from build123d import *

# Parameters (mm, degrees)
SKETCH1_W           = 54
SKETCH1_H           = 59
SKETCH1_W_2         = 40
SKETCH1_H_2         = 52
BOSS_EXTRUDE1_DEPTH = 12
SKETCH2_R           = 1.85
CUT_EXTRUDE1_DEPTH  = 10
SKETCH3_R           = 1.85
CUT_EXTRUDE2_DEPTH  = 10
SKETCH4_W           = 54
SKETCH4_H           = 12
CUT_EXTRUDE4_DEPTH  = 40
SKETCH5_W           = 7
SKETCH5_H           = 12
CUT_EXTRUDE5_DEPTH  = 40
SKETCH6_W           = 12
SKETCH6_H           = 12
BOSS_EXTRUDE2_DEPTH = 5
SKETCH7_R           = 2.6
CUT_EXTRUDE6_DEPTH  = 2.4


with BuildPart() as part:
    # Sketch1 → Boss-Extrude1 (new body)
    with BuildSketch(Plane.XY):
        with Locations((27, 29.5)):
            Rectangle(SKETCH1_W, SKETCH1_H)
        with Locations((27, 29.5)):
            Rectangle(SKETCH1_W_2, SKETCH1_H_2, mode=Mode.SUBTRACT)
    extrude(amount=BOSS_EXTRUDE1_DEPTH)

    # Sketch2 → Cut-Extrude1 (cut)
    with BuildSketch(Plane(origin=(0, 59, 0), x_dir=(1, 0, 0), z_dir=(0, 1, 0))):
        with Locations(Location((13, -9.7, 0), (0, 0, 180))):
            Circle(SKETCH2_R)
        with Locations(Location((41, -9.7, 0), (0, 0, 180))):
            Circle(SKETCH2_R)
        with Locations(Location((27, -9.7, 0), (0, 0, 180))):
            Circle(SKETCH2_R)
    extrude(amount=-CUT_EXTRUDE1_DEPTH, mode=Mode.SUBTRACT)

    # Sketch3 → Cut-Extrude2 (cut)
    with BuildSketch(Plane.XZ):
        with Locations(Location((12.75, 6, 0), (0, 0, 270))):
            Circle(SKETCH3_R)
        with Locations(Location((41.25, 6, 0), (0, 0, 90))):
            Circle(SKETCH3_R)
    extrude(amount=-CUT_EXTRUDE2_DEPTH, mode=Mode.SUBTRACT)

    # Sketch4 → Cut-Extrude4 (cut)
    with BuildSketch(Plane.XZ):
        with Locations((27, 6)):
            Rectangle(SKETCH4_W, SKETCH4_H)
    extrude(amount=-CUT_EXTRUDE4_DEPTH, mode=Mode.SUBTRACT)

    # Sketch5 → Cut-Extrude5 (cut)
    with BuildSketch(Plane.XZ.offset(-40)):
        with Locations((3.5, 6)):
            Rectangle(SKETCH5_W, SKETCH5_H)
        with Locations((50.5, 6)):
            Rectangle(SKETCH5_W, SKETCH5_H)
    extrude(amount=-CUT_EXTRUDE5_DEPTH, mode=Mode.SUBTRACT)

    # Sketch6 → Boss-Extrude2 (add)
    with BuildSketch(Plane(origin=(47, 0, 0), x_dir=(0, 0, -1), z_dir=(1, 0, 0))):
        with Locations((-6, 53)):
            Rectangle(SKETCH6_W, SKETCH6_H)
    boss_extrude2 = extrude(amount=BOSS_EXTRUDE2_DEPTH)

    # Mirror1: Boss-Extrude2 across plane
    add(boss_extrude2.mirror(Plane.ZY.offset(-27)))

    # Sketch7 → Cut-Extrude6 (cut)
    with BuildSketch(Plane.ZY.offset(-2)):
        with Locations((6, 54)):
            Circle(SKETCH7_R)
    cut_extrude6 = extrude(amount=-CUT_EXTRUDE6_DEPTH, mode=Mode.SUBTRACT)

    # Mirror2: Cut-Extrude6 across plane
    add(cut_extrude6.mirror(Plane.ZY.offset(-27)), mode=Mode.SUBTRACT)


solid = part.part
For this review, take the finished solid that the model builds, in its own axes (mm). A direction names the side the tool comes from. Round coordinates to 2 decimals unless told otherwise and drop trailing zeros. Order: outer loops, then holes, each group sorted by start corner. A loop starts at its lowest first (then second) coordinate and runs counter-clockwise, first axis right, second up. Notation, with made-up numbers: M -38,49 L 3,49 A31 ccw 3,79 Z; hole C -22,16 d7. An arc over 180 degrees is marked long. Use a Markdown table: item, result. Add a question column.
Item 1: Add section A-A, the plane z = 9.7. Give the boundary of the cut face in (x, y), then the cut area to 3 significant figures.
Item 2: Add section D-D, the plane z = 1.5. Give the boundary of the cut face in (x, y), then the cut area to 3 significant figures.
Item 3: Tool access review of faces 4 (the cylindrical face through (50.82, 51.46, 5.44)), 5 (the flat face through (7, 51, 6)), 6 (the flat face through (4.4, 54, 6)): name each direction out of +Z, -Z, +X, -X, +Y, -Y from which nothing blocks a thin tool from reaching the whole face with its end or side.
Item 4: Insertion check: pin 1 (3 mm diameter, centred on x = 27, z = 9.7, fed in from +Y); pin 2 (1.6 mm diameter, centred on y = 55, z = 7, fed in from -X). Each pin has a flat end and moves straight along its axis. Give the tip position at first contact, or say it passes through.
Item 5: To check wall thickness, follow line 1 along X through (y, z) = (55, 7.25); line 2 along X through (y, z) = (52.5, 9.5); line 3 along Y through (x, z) = (50.95, 6). State the ranges of each line that lie inside material, in increasing order.
Item 6: Add section B-B, the plane x = 41. Give the boundary of the cut face in (y, z).
Item 7: Mouldability with a two-part tool opening along Y and no side actions: class faces 1 (the flat face through (27, 56, 12)), 2 (the flat face through (5, 47, 6)), 3 (the flat face through (49.6, 54, 6)) as released by +Y, released by -Y, zero draft, split by the parting line, or undercut.
Item 8: Add section C-C, the plane y = 49. Give the boundary of the cut face in (x, z).
Geometry results:
| question | item | result |
|---|---|---|
| 1 | outline | M 2,47 L 7,47 L 7,55.5 L 11.15,55.5 L 11.15,59 L 2,59 Z; M 14.85,55.5 L 25.15,55.5 L 25.15,59 L 14.85,59 Z; M 28.85,55.5 L 39.15,55.5 L 39.15,59 L 28.85,59 Z; M 42.85,55.5 L 47,55.5 L 47,47 L 52,47 L 52,59 L 42.85,59 Z |
| 1 | area | 221 mm² |
| 2 | outline | M 2,47 L 7,47 L 7,55.5 L 47,55.5 L 47,47 L 52,47 L 52,59 L 2,59 Z |
| 2 | area | 260 mm² |
| 3 | face 4 | +X |
| 3 | face 5 | +Z, -Z, -Y |
| 3 | face 6 | -X |
| 4 | pin 1 | passes through |
| 4 | pin 2 | stops at x = 4.4 |
| 5 | line 1 | x = 4.4 to 7, 47 to 49.6 |
| 5 | line 2 | x = 2 to 7, 47 to 52 |
| 5 | line 3 | y = 47 to 51.4, 56.6 to 59 |
| 6 | outline | M 55.5,0 L 59,0 L 59,7.85 L 55.5,7.85 Z; M 55.5,11.55 L 59,11.55 L 59,12 L 55.5,12 Z |
| 7 | face 1 | zero draft |
| 7 | face 2 | released by -Y |
| 7 | face 3 | undercut |
| 8 | outline | M 2,0 L 7,0 L 7,12 L 2,12 Z; M 47,0 L 52,0 L 52,12 L 47,12 Z |
